Autodesk Inventor part; units mm, degrees
ref_plane "YZ Plane" through (0, 0, 0) normal (1, 0, 0) x (0, 1, 0)
ref_plane "XZ Plane" through (0, 0, 0) normal (0, 1, 0) x (-1, 0, 0)
ref_plane "XY Plane" through (0, 0, 0) normal (0, 0, 1) x (1, 0, 0)
sketch "Szkic3" plane through (0, 0, 0) normal (0, 1, 0) x (-1, 0, 0)
  line L0 (3, 4) -> (-3, 4)
  line L1 (-3, 4) -> (-3, -4)
  line L2 (-3, -4) -> (3, -4)
  line L3 (3, -4) -> (3, 4)
  line L4 (3, 4) -> (-3, -4) construction
  line L5 (-3, 4) -> (3, -4) construction
  point P0 (0, 0)
  dimension "d8" = 6
  dimension "d9" = 8
extrude "Wyciągnięcie proste2" add sketch "Szkic3" along normal blind 11
sketch "Szkic4" plane through (-3, 0, 4) normal (0, 0, 1) x (1, 0, 0)
  circle A0 centre (3, 3.5) radius 2.5
  line L0 (6, 0) -> (6, 11)
  line L1 (0, 0) -> (0, 11)
  circle A1 centre (3, 8.6) radius 1.6
  point P0 (3, 0)
  dimension "d12" = 5
  dimension "d13" = 3
  dimension "d14" = 3
  dimension "d15" = 3.5
  dimension "d16" = 3.2
  dimension "d17" = 5.1
extrude "Wyciągnięcie proste3" cut sketch "Szkic4" against normal up to next contours A1
extrude "Wyciągnięcie proste4" cut sketch "Szkic4" against normal up to next draft -5 contours A0
sketch "Szkic5" plane through (0, 0, 0) normal (0, -1, 0) x (1, 0, 0)
  circle A0 centre (0, 0) radius 1.2
  dimension "d22" = 2.4
extrude "Wyciągnięcie proste5" add sketch "Szkic5" along normal blind 1.5 draft -5
fillet "Fillet2" radius 3 2 edges at (-3, 11, 0) (3, 11, 0)
equation "\"d14\" = d13"
properties part number "mocowanieDiod"
The listing builds one solid part. Answer for the finished solid, in the listing's coordinates (mm). A direction names the side the tool comes from. Give positions to 0.01 mm unless a question says otherwise; leave off trailing zeros. Loops run counter-clockwise (first coordinate to the right, second up) from the corner with the lowest first, then second, coordinate; pieces in that order, holes last. Notation, with made-up numbers: (86, -19) - (107, -19) arc R19 ccw to (107, -8) - close; hole circle Ø4 at (-23, 88.5). An arc over 180 degrees is marked (long way). Return JSON: item names as keys, results as strings. Group by question number.
1. Find section D-D (y = 8.6). Write down the section's boundary in (x, z).
2. Find section A-A (y = 3.5). Write down the section's boundary in (x, z).
3. Which of the six approach directions +Z, -Z, +X, -X, +Y, -Y give full straight-line access (tool end or side, diameter ignored) to faces 1 (the flat face through (-0.6, 5.4, -4)), 2 (the flat face through (1.4, 0, 0.1))?
4. Given pin 1 Ø1.5 at (x, z) = (1.5, -1.5) entering from +Y; pin 2 Ø1.5 at (x, z) = (2, -3) entering from -Y, each flat-ended and moving along its own axis, determine where each tip first touches the part or whether it passes through.
5. Determine the mould class of faces 3 (the conical face through (-0.89, -0.91, 0.68)), 4 (the flat face through (3, 4, 0)), 5 (the cylindrical face through (-0.208, 10.186, 0.056)) for opening direction X: pulls with the +X half, pulls with the -X half, needs draft (parallel to the pull), parting line crosses it, or undercut.
6. Find section B-B (z = 2.5). State how many separate pieces and enclosed holes the cut face has, then the cut area to 3 significant figures.
7. Straight lines are drawn through the part: line 1 (Y direction, x = 0.25, z = -2.25); line 2 (Y direction, x = 1.2, z = 0.75); line 3 (X direction, y = 10, z = 0). For each, find the intervals that lie inside material, in ascending order. Write a range as [from, to].
Verdict:
{
 "1": {"outline": "(-2.94, -4) - (-1.6, -4) - (-1.6, 4) - (-2.94, 4) - close; (1.6, -4) - (2.94, -4) - (2.94, 4) - (1.6, 4) - close"},
 "2": {"outline": "(-3, -4) - (-1.8, -4) - (-2.5, 4) - (-3, 4) - close; (1.8, -4) - (3, -4) - (3, 4) - (2.5, 4) - close"},
 "3": {"face 1": "-Z, +X, -X, +Y, -Y", "face 2": "-Y"},
 "4": {"pin 1": "stops at y = 10.9", "pin 2": "stops at y = 0"},
 "5": {"face 3": "parting line crosses it", "face 4": "pulls with the +X half", "face 5": "undercut"},
 "6": {"separate pieces": "1", "enclosed holes": "2", "area": "36.5 mm^2"},
 "7": {"line 1": "y = [0, 1.56], [5.44, 7.02], [10.18, 10.99]", "line 2": "y = [0, 1.64], [5.36, 7.54], [9.66, 10.75]", "line 3": "x = [-2.24, -0.77], [0.77, 2.24]"}
}
